Can you work these out from the model? Positions are in its coordinate system, mm. A direction names the side the tool comes from. Give positions to 0.01 mm unless a question says otherwise; leave off trailing zeros. Order: outer loops, then holes, each group sorted by start corner. A loop starts at its lowest first (then second) coordinate and runs counter-clockwise, first axis right, second up. Notation, with made-up numbers: (9.25, 60.5) - (33.25, 60.5) arc R28 cw to (33.25, 92.5) - close; hole circle Ø2 at (-38.5, -22). An arc over 180 degrees is marked (long way). Answer as CSV lines item,"result".
```python
from build123d import *

# Parameters (mm, degrees)
F1_DEPTH = 29
F2_W     = 15
F2_H     = 18.9897948557
F3_DEPTH = 58.001
F4_SIZE  = 4
F6_DEPTH = 3
F7_R     = 2.25
F8_DEPTH = 58.001
F9_R     = 2


with BuildPart() as f1:
    # F0 (on Front) → F1 (new body, symmetric)
    with BuildSketch(Plane.XZ):
        with BuildLine():
            Line((10, -20), (10, -48.9897948557))
            ThreePointArc((10, -48.9897948557), (31.4520402548, -38.8686141226), (45.8257569496, -20))
            Line((45.8257569496, -20), (10, -20))
        make_face()
    extrude(amount=F1_DEPTH, both=True)

    # F2 (on face) → F3 (cut, through all)
    with BuildSketch(Plane.XZ.offset(29)):
        with Locations((17.5, -29.4948974278)):
            Rectangle(F2_W, F2_H)
    extrude(amount=-F3_DEPTH, mode=Mode.SUBTRACT)

    # F4
    f4_edges = [f1.edges().sort_by_distance(p)[0] for p in [
        (25, 0, -38.989795),
    ]]
    chamfer(f4_edges, length=F4_SIZE)

    # F5 (on face) → F6 (cut)
    with BuildSketch(Plane(origin=(10, 0, 0), x_dir=(0, -1, 0), z_dir=(-1, 0, 0))):
        with BuildLine():
            Line((-16, -38.9897948557), (-16, -44))
            ThreePointArc((-16, -44), (-14.1480502971, -46.7716385975), (-10.8786796564, -46.1213203436))
            Line((-10.8786796564, -46.1213203436), (-3.7471541685, -38.9897948557))
            Line((-3.7471541685, -38.9897948557), (-16, -38.9897948557))
        make_face()
        with BuildLine():
            Line((10, -38.9897948557), (10, -44))
            ThreePointArc((10, -44), (11.8519497029, -46.7716385975), (15.1213203436, -46.1213203436))
            Line((15.1213203436, -46.1213203436), (22.2528458315, -38.9897948557))
            Line((22.2528458315, -38.9897948557), (10, -38.9897948557))
        make_face()
    extrude(amount=-F6_DEPTH, mode=Mode.SUBTRACT)

    # F7 (on face) → F8 (cut, through all)
    with BuildSketch(Plane.XZ.offset(29)):
        with Locations((32, -27)):
            Circle(F7_R)
    extrude(amount=-F8_DEPTH, mode=Mode.SUBTRACT)

    # F9
    f9_edges = [f1.edges().sort_by_distance(p)[0] for p in [
        (25, 0, -20),
        (25, 0, -34.989795),
        (21, 0, -38.989795),
    ]]
    fillet(f9_edges, radius=F9_R)


solid = f1.part
```
1) I need wall thicknesses on line 1 along Z through (x, y) = (32, 7); line 2 along Z through (x, y) = (33, -1.5); line 3 along Z through (x, y) = (43, 22.5). Which ranges of each line are inside material? Lowest first, please. Write a range as [from, to].
Answer block:
line 1,"[-38.42, -29.25], [-24.75, -20]"
line 2,"[-37.56, -29.02], [-24.98, -20]"
line 3,"[-25.51, -20]"
2) I want a section at B-B on x = 32. Write out the boundary of the cut face in (y, z), plus the area to 3 significant figures.
Answer block:
outline,"(-29, -38.42) - (29, -38.42) - (29, -29.25) - (-29, -29.25) - close; (-29, -24.75) - (29, -24.75) - (29, -20) - (-29, -20) - close"
area,"807 mm2"
3) I want a section at C-C on z = -27.75. Write out the boundary of the cut face in (x, y), plus the area to 3 significant figures.
Answer block:
outline,"(25, -29) - (29.88, -29) - (29.88, 29) - (25, 29) - close; (34.12, -29) - (41.59, -29) - (41.59, 29) - (34.12, 29) - close"
area,"716 mm2"
4) I want a section at D-D on y = -13.5. Write out the boundary of the cut face in (x, z).
Answer block:
outline,"(10, -48.99) arc R50 ccw to (45.83, -20) - (27, -20) arc R2 ccw to (25, -22) - (25, -34.16) arc R2 cw to (24.41, -35.58) - (21.59, -38.4) arc R2 cw to (20.17, -38.99) - (13, -38.99) - (13, -46.96) - (10, -46.96) - close; hole circle Ø4.5 at (32, -27)"
5) I'm going to push flat-ended pins straight in: P1, Ø8, axis at x = 16.5, y = -5.5, coming from the +Z side; P2, Ø3, axis at x = 16.5, y = 5.5, coming from the -Z side; P3, Ø12, axis at x = 20.5, y = -5, coming from the -Z side; P4, Ø9, axis at y = 9.5, z = -43, coming from the -X side. Where does each tip first touch, or does it pass through?
Answer block:
P1,"z = -38.96"
P2,"z = -47.7"
P3,"z = -47.85"
P4,"x = 10"
6) I want a section at A-A on y = -4. Write out the boundary of the cut face in (x, z).
Answer block:
outline,"(10, -48.99) arc R50 ccw to (45.83, -20) - (27, -20) arc R2 ccw to (25, -22) - (25, -34.16) arc R2 cw to (24.41, -35.58) - (21.59, -38.4) arc R2 cw to (20.17, -38.99) - (10, -38.99) - close; hole circle Ø4.5 at (32, -27)"
7) Which directions (+Z, -Z, +X, -X, +Y, -Y) give clear straight access to the entire face, cutting with the end or side of a thin tool? Please do faces 1 (the flat face through (25, 0, -28)), 2 (the cylindrical face through (31.19, -0.41, -39.08)), 3 (the flat face through (11, -10, -41)).
Answer block:
face 1,"+Z, -X, +Y, -Y"
face 2,"-Z, +X, +Y, -Y"
face 3,"+Z, -X"
